Geometry: final body of the model. Coordinates: model frame, mm. Round coordinates to 2 decimals unless told otherwise and drop trailing zeros. Loops run counter-clockwise (first coordinate to the right, second up) from the corner with the lowest first, then second, coordinate; pieces in that order, holes last. Notation, with made-up numbers: (-4, 35.25) -> (48, 35.25) arc R28 cw to (48, 61.25) -> close; hole circle Ø2 at (82, -1.75). An arc over 180 degrees is marked (long way). Answer in a Markdown table with one row per item.
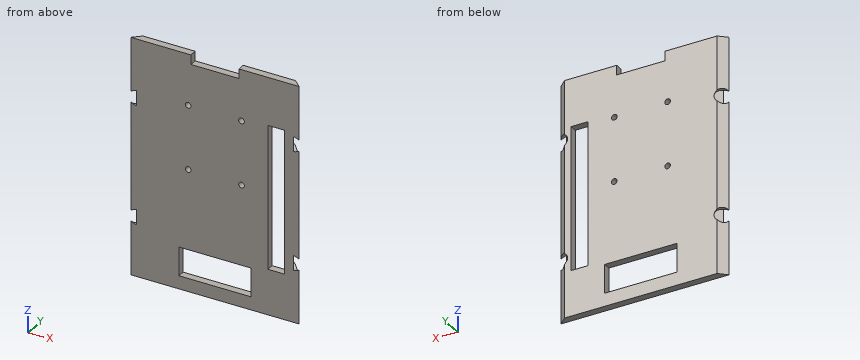
```python
from build123d import *

# Parameters (mm, degrees)
BOSS_EXTRUDE1_DEPTH = 125.73
SKETCH3_W           = 25.4
SKETCH3_H           = 5.08
CUT_EXTRUDE1_DEPTH  = 134.393493158
SKETCH5_W           = 8.89
SKETCH5_H           = 76.2
CUT_EXTRUDE3_DEPTH  = 134.393493158
SKETCH6_W           = 38.1
SKETCH6_H           = 15.24
CUT_EXTRUDE4_DEPTH  = 134.393493158
SKETCH7_R           = 4.0005
CUT_EXTRUDE5_DEPTH  = 2
SKETCH8_R           = 4.0005
CUT_EXTRUDE6_DEPTH  = 2
SKETCH9_R           = 1.5
CUT_EXTRUDE8_DEPTH  = 134.393493158


with BuildPart() as part:
    # Sketch1 → Boss-Extrude1 (new body)
    with BuildSketch(Plane.XY):
        Polygon((-40.203883769, 5.937788296), (40.203883769, 5.937788296), (44.399042974, 2.127788296), (-44.399042974, 2.127788296), align=None)
    extrude(amount=BOSS_EXTRUDE1_DEPTH)

    # Sketch3 → Cut-Extrude1 (cut, through all)
    with BuildSketch(Plane.XZ.offset(-2.127788296)):
        with Locations((0, 123.19)):
            Rectangle(SKETCH3_W, SKETCH3_H)
    extrude(amount=-CUT_EXTRUDE1_DEPTH, mode=Mode.SUBTRACT)

    # Sketch5 → Cut-Extrude3 (cut, through all)
    with BuildSketch(Plane.XZ.offset(-2.127788296)):
        with Locations((32.334042974, 62.23)):
            Rectangle(SKETCH5_W, SKETCH5_H)
    extrude(amount=-CUT_EXTRUDE3_DEPTH, mode=Mode.SUBTRACT)

    # Sketch6 → Cut-Extrude4 (cut, through all)
    with BuildSketch(Plane.XZ.offset(-2.127788296)):
        with Locations((0, 14.553010533)):
            Rectangle(SKETCH6_W, SKETCH6_H)
    extrude(amount=-CUT_EXTRUDE4_DEPTH, mode=Mode.SUBTRACT)

    # Sketch7 → Cut-Extrude5 (cut)
    with BuildSketch(Plane(origin=(21.127225221, 23.263011377, 0), x_dir=(0.7402720771062569, -0.6723074087475075, 0), z_dir=(0.6723074087475075, 0.7402720771062569, 0))):
        with Locations((28.603318705, -94.361)):
            Circle(SKETCH7_R)
        with Locations((28.603318705, -31.369)):
            Circle(SKETCH7_R)
    extrude(amount=-CUT_EXTRUDE5_DEPTH, mode=Mode.SUBTRACT)

    # Sketch8 → Cut-Extrude6 (cut)
    with BuildSketch(Plane(origin=(-21.127225221, 23.263011377, 0), x_dir=(0.7402720771062569, 0.6723074087475075, 0), z_dir=(-0.6723074087475075, 0.7402720771062569, 0))):
        with Locations((-28.603318705, -31.369)):
            Circle(SKETCH8_R)
        with Locations((-28.603318705, -94.361)):
            Circle(SKETCH8_R)
    extrude(amount=-CUT_EXTRUDE6_DEPTH, mode=Mode.SUBTRACT)

    # Sketch9 → Cut-Extrude8 (cut, through all)
    with BuildSketch(Plane(origin=(0, 5.937788296, 0), x_dir=(1, 0, 0), z_dir=(0, 1, 0))):
        with Locations(Location((13.978116231, -98.601597848, 0), (0, 0, 270))):
            Circle(SKETCH9_R)
        with Locations(Location((-14.121883769, -98.601597848, 0), (0, 0, 270))):
            Circle(SKETCH9_R)
        with Locations(Location((-14.121883769, -64.601597848, 0), (0, 0, 270))):
            Circle(SKETCH9_R)
        with Locations(Location((13.978116231, -64.601597848, 0), (0, 0, 270))):
            Circle(SKETCH9_R)
    extrude(amount=-CUT_EXTRUDE8_DEPTH, mode=Mode.SUBTRACT)


solid = part.part
```
Item 1: Cut plane D-D (z = 107). Output: boundary loops of the cut face in (x, y).
Answer:
| item | result |
|---|---|
| outline | (-44.4, 2.13) -> (44.4, 2.13) -> (40.2, 5.94) -> (-40.2, 5.94) -> close |
Item 2: Pin query (flat end, axial travel): pin 1 Ø1.1 at (y, z) = (4.5, 13.5) entering from -X; pin 2 Ø1.9 at (x, y) = (5, 4) entering from +Z; pin 3 Ø1.9 at (y, z) = (4, 122.5) entering from +X; pin 4 Ø1.8 at (x, z) = (13.98, 64.6) entering from +Y. Return the tip coordinate at first contact, or that it passes through.
Answer:
| item | result |
|---|---|
| pin 1 | stops at x = -42.39 |
| pin 2 | stops at z = 120.65 |
| pin 3 | stops at x = 43.38 |
| pin 4 | passes through |
Item 3: Cut plane B-B (x = 33.5). Output: boundary loops of the cut face in (y, z), then the cut area to 3 significant figures.
Answer:
| item | result |
|---|---|
| outline | (2.13, 0) -> (5.94, 0) -> (5.94, 24.13) -> (2.13, 24.13) -> close; (2.13, 100.33) -> (5.94, 100.33) -> (5.94, 125.73) -> (2.13, 125.73) -> close |
| area | 189 mm² |
Item 4: Line query: probe 1 along Z at (x, y) = (-39, 4.6); probe 2 along Z at (x, y) = (-6, 5.55); probe 3 along Z at (x, y) = (29.5, 4.65). Output: solid intervals per line, ascending. Write a range as [from, to].
Answer:
| item | result |
|---|---|
| probe 1 | z = [0, 28.54], [34.2, 91.53], [97.19, 125.73] |
| probe 2 | z = [0, 6.93], [22.17, 120.65] |
| probe 3 | z = [0, 24.13], [100.33, 125.73] |
Item 5: Cut plane A-A (z = 18). Output: boundary loops of the cut face in (x, y).
Answer:
| item | result |
|---|---|
| outline | (-44.4, 2.13) -> (-19.05, 2.13) -> (-19.05, 5.94) -> (-40.2, 5.94) -> close; (19.05, 2.13) -> (44.4, 2.13) -> (40.2, 5.94) -> (19.05, 5.94) -> close |
Item 6: Cut plane C-C (y = 3.55). Count the separate pieces of the cut face and the enclosed holes in it, then the cut area to 3 significant figures.
Answer:
| item | result |
|---|---|
| separate pieces | 1 |
| enclosed holes | 6 |
| area | 9,260 mm² |
